Geometry: final body of the model. Coordinates: model frame, mm. A direction names the side the tool comes from. Give positions to 0.01 mm unless a question says otherwise; leave off trailing zeros. Write each loop counter-clockwise with the first axis right and the second up, starting at its lowest first coordinate (ties: lowest second). Pieces come first, ordered by that corner, then holes.
Autodesk Inventor part; units mm, degrees
ref_plane "Work Plane1" through (2.85, -21, 0) normal (0, 0, -1) x (-1, 0, 0)
ref_plane "YZ Plane" through (0, 0, 0) normal (1, 0, 0) x (0, 1, 0)
ref_plane "XZ Plane" through (0, 0, 0) normal (0, 1, 0) x (-1, 0, 0)
sketch "Sketch1" plane through (0, 0, 0) normal (1, 0, 0) x (0, 1, 0)
  line L0 (21, 41.5) -> (-21, 41.5)
  line L1 (-21, 41.5) -> (-21, -41.5)
  line L2 (-21, -41.5) -> (21, -41.5)
  line L3 (21, -41.5) -> (21, 41.5)
  point P0 (0, 0)
  dimension "d0" = 83
  dimension "d1" = 41.5
  dimension "d2" = 42
  dimension "d3" = 21
extrude "Extrusion1" add sketch "Sketch1" along normal blind 2.85
sketch "Sketch3" plane through (2.85, 0, 0) normal (1, 0, 0) x (0, 0, -1)
  line L0 (41.5, 21) -> (-41.5, 21)
  line L1 (-41.5, 21) -> (2.5, 21)
  line L2 (2.5, 21) -> (2.5, 19)
  line L3 (2.5, 19) -> (-41.5, 19)
  line L4 (-41.5, 19) -> (-41.5, 21)
  line L5 (-41.5, -21) -> (41.5, -21)
  line L6 (41.5, -21) -> (3.5, -21)
  line L7 (3.5, -21) -> (3.5, -19)
  line L8 (3.5, -19) -> (41.5, -19)
  line L9 (41.5, -19) -> (41.5, -21)
  line L10 (41.5, -21) -> (41.5, 21)
  line L11 (41.5, 21) -> (-41.5, 21)
  line L12 (-41.5, 21) -> (-41.5, -21)
  line L13 (-41.5, -21) -> (41.5, -21)
  point P0 (0, 0)
  point P1 (41.5, 21)
  dimension "d12" = 44
  dimension "d13" = 2
  dimension "d14" = 38
  dimension "d15" = 2
extrude "Extrusion3" add sketch "Sketch3" along normal blind 3 contours L10 L8 L7 L5 L12 L3 L2 L0
sketch "Sketch4" plane through (0, 21, 41.5) normal (0, 1, 0) x (1, 0, 0)
  line L0 (0, 83) -> (0, 0)
  line L1 (2.85, 44) -> (5.85, 44)
  line L2 (0, 83) -> (5.85, 83)
  line L3 (5.85, 83) -> (5.85, 44)
  line L4 (5.85, 44) -> (0, 44)
  line L5 (0, 44) -> (0, 83)
  point P0 (0, 41.5)
extrude "Extrusion4" cut sketch "Sketch4" against normal blind 7.5
sketch "Sketch5" plane through (0, -21, 41.5) normal (0, 0, 1) x (1, 0, 0)
  circle A0 centre (17.475, 18) radius 6.625
  circle A1 centre (17.475, 18) radius 11.625
  line L0 (5.85, 40) -> (5.85, 0)
  line L1 (5.85, 2) -> (5.85, 34.5)
  line L2 (2.85, 40) -> (5.85, 40)
  line L3 (17.475, 6.375) -> (5.85, 6.375)
  line L4 (28.3902, 22) -> (12.1938, 22)
  line L5 (28.3902, 14) -> (12.1938, 14)
  line L6 (17.475, 29.625) -> (5.85, 29.625)
  line L7 (17.475, 18) -> (5.85, 18)
  line L8 (0, 0) -> (5.85, 0)
  point P0 (0, 21)
  point P1 (22.7562, 14)
  point P2 (22.7562, 22)
  dimension "d20" = 13.25
  dimension "d21" = 5
  dimension "d30" = 18
  dimension "d31" = 4
  dimension "d32" = 4
extrude "Extrusion5" add sketch "Sketch5" against normal blind 5 contours A0 L7 A1 L4 | L5 A1 L7 A0 | A1 L0 L6 | L3 L0 A1
fillet "Fillet3" radius 3 3 edges at (5.85, -14.625, 39) (5.85, -3, 36.5) (5.85, 8.625, 39)
ref_plane "Work Plane1" through (2.85, -21, 0) normal (0, 0, -1) x (-1, 0, 0)
mirror "Mirror1" about plane through (2.85, -21, 0) normal (0, 0, -1) of "Extrusion5", "Fillet3"
sketch "Sketch6" plane through (0, -21, 36.5) normal (0, 0, -1) x (-1, 0, 0)
  line L0 (-8.85, 29.625) -> (-8.85, 6.375)
  line L1 (-8.85, 29.625) -> (-17.475, 29.625)
  arc A0 (-17.475, 29.625) -> (-28.3902, 22) centre (-17.475, 18) ccw
  line L2 (-28.3902, 22) -> (-22.7562, 22)
  arc A1 (-22.7562, 14) -> (-22.7562, 22) centre (-17.475, 18) ccw
  line L3 (-22.7562, 14) -> (-28.3902, 14)
  arc A2 (-28.3902, 14) -> (-17.475, 6.375) centre (-17.475, 18) ccw
  line L4 (-17.475, 6.375) -> (-8.85, 6.375)
  line L5 (-17.475, 18) -> (-23.2875, 28.0675)
  arc A3 (-17.475, 29.625) -> (-28.3902, 22) centre (-17.475, 18) ccw
  line L6 (-17.475, 18) -> (-5.85, 18) construction
  line L7 (-17.475, 18) -> (-23.2875, 7.9325)
  arc A4 (-28.3902, 14) -> (-17.475, 6.375) centre (-17.475, 18) ccw
  line L8 (-17.475, 18) -> (-5.85, 18) construction
  point P0 (0, 21)
  point P1 (-20.7875, 23.7374)
  point P2 (-20.7875, 12.2626)
  dimension "d33" = 120
  dimension "d42" = 120
extrude "Extrusion6" cut sketch "Sketch6" against normal blind 13.5 contours A2 L3 A1 L7
sketch "Sketch7" plane through (2.85, -21, -41.5) normal (0, 0, -1) x (-1, 0, 0)
  line L0 (2.85, 34.5) -> (-3, 34.5)
  line L1 (-3, 32.625) -> (-3, 34.5)
  arc A0 (-6, 29.625) -> (-3, 32.625) centre (-6, 32.625) ccw
  line L2 (-14.625, 29.625) -> (-6, 29.625)
  arc A1 (-14.625, 29.625) -> (-25.5402, 22) centre (-14.625, 18) ccw
  line L3 (-19.9062, 22) -> (-25.5402, 22)
  arc A2 (-19.9062, 14) -> (-19.9062, 22) centre (-14.625, 18) ccw
  line L4 (-25.5402, 14) -> (-19.9062, 14)
  arc A3 (-25.5402, 14) -> (-14.625, 6.375) centre (-14.625, 18) ccw
  line L5 (-6, 6.375) -> (-14.625, 6.375)
  arc A4 (-3, 3.375) -> (-6, 6.375) centre (-6, 3.375) ccw
  line L6 (-3, 2) -> (-3, 3.375)
  line L7 (0, 2) -> (-3, 2)
  line L8 (0, 0) -> (0, 2)
  line L9 (2.85, 0) -> (0, 0)
  line L10 (2.85, 0) -> (2.85, 34.5)
  arc A5 (-14.625, 29.625) -> (-25.5402, 22) centre (-14.625, 18) ccw
  line L11 (-19.9062, 22) -> (-25.5402, 22)
  line L12 (-14.625, 18) -> (-20.4375, 7.9325)
  arc A6 (-25.5402, 14) -> (-14.625, 6.375) centre (-14.625, 18) ccw
  line L13 (-14.625, 18) -> (-3, 18) construction
  line L14 (-25.5402, 14) -> (-19.9062, 14)
  arc A7 (-19.9062, 14) -> (-19.9062, 22) centre (-14.625, 18) ccw
  line L15 (-17.9375, 12.2626) -> (-22.711, 14)
  line L16 (-17.9375, 12.2626) -> (-12.8576, 12.2626) construction
  point P0 (2.85, 21)
  dimension "d43" = 120
  dimension "d44" = 160
extrude "Extrusion7" cut sketch "Sketch7" against normal blind 11.5 contours L15 L4 A2
sketch "Sketch8" plane through (0, 13.5, 41.5) normal (0, 1, 0) x (1, 0, 0)
  line L0 (2.85, 44) -> (0, 44)
  line L1 (0, 83) -> (5.85, 83)
  line L2 (2.85, 44) -> (5.85, 44)
  line L3 (5.85, 44) -> (5.85, 83)
  line L4 (5.85, 83) -> (2.85, 83)
  line L5 (2.85, 83) -> (2.85, 44)
  point P0 (0, 41.5)
extrude "Extrusion8" add sketch "Sketch8" along normal up to surface (5.5 mm away)
equation "\"d32\" = d31"
properties part number "Lid"
Item 1: Section C-C, the plane y = 15.5. Return the cut outline in (x, z), plus the area to 3 significant figures.
Found:
outline: (0, -2.5) - (2.85, -2.5) - (2.85, -41.5) - (5.85, -41.5) - (5.85, 41.5) - (0, 41.5) - close
area: 374 mm2
Item 2: Reachability of faces 5 (the face through (23.14, -7.88, -39.03)), 6 (the face through (1, 17, -2.5)), 7 (the face through (26, 1, -39)) from +Z, -Z, +X, -X, +Y, -Y: full face, straight path, thin tool, end or side. Return the list, or none.
Found:
face 5: +Z, -Z
face 6: -Z, -X, +Y
face 7: +Z, -Z, +X
Item 3: Pin query (flat end, axial travel): pin 1 Ø3 at (x, z) = (8, 19) entering from -Y; pin 2 Ø0.9 at (x, y) = (1.5, 16) entering from -Z; pin 3 Ø12 at (x, z) = (10, -28) entering from -Y; pin 4 Ø2 at (y, z) = (16, -29) entering from -X. Return the tip coordinate at first contact, or that it passes through.
Found:
pin 1: passes through
pin 2: stops at z = -2.5
pin 3: stops at y = -19
pin 4: stops at x = 2.85
Item 4: Line query: L1, parallel to Z at x = 12.75, y = -10.5; L2, parallel to X at y = -3, z = 37.75; L3, parallel to X at y = 6, z = -2. Output: solid intervals per line, ascending.
Found:
L1: z = -41.5 to -36.5, 36.5 to 41.5
L2: x = 0 to 10.85
L3: x = 0 to 5.85
Item 5: Section B-B, the plane y = -3. Return the cut outline in (x, z), plus the area to 3 significant figures.
Found:
outline: (0, -41.5) - (10.85, -41.5) - (10.85, -36.5) - (8.85, -36.5) arc R3 cw to (5.85, -33.5) - (5.85, 33.5) arc R3 cw to (8.85, 36.5) - (10.85, 36.5) - (10.85, 41.5) - (0, 41.5) - close
area: 539 mm2
Item 6: Section D-D, the plane z = 5.5. Return the cut outline in (x, y), plus the area to 3 significant figures.
Found:
outline: (0, -21) - (5.85, -21) - (5.85, 19) - (2.85, 19) - (2.85, 21) - (0, 21) - close
area: 240 mm2
Item 7: Section A-A, the plane z = -8. Return the cut outline in (x, y).
Found:
outline: (0, -21) - (2.85, -21) - (2.85, -19) - (5.85, -19) - (5.85, 19) - (2.85, 19) - (2.85, 13.5) - (0, 13.5) - close
Item 8: Pull-direction query (Y, two-part tool) for faces 1 (the face through (13, 8.625, -39)), 2 (the face through (22.02, -10.87, 38.97)), 3 (the face through (12, -8, -36.5)), 4 (the face through (27, -7, -39)); classes: +Y half, -Y half, draft (parallel to the pull), parting line (faces both ways), or undercut.
Found:
face 1: +Y half
face 2: undercut
face 3: draft
face 4: undercut
